Can you work these out from the model? Positions are in its coordinate system, mm. A direction names the side the tool comes from. Coordinates: 2 decimals unless noted, no trailing zeros. Order: outer loops, then holes, each group sorted by start corner. A loop starts at its lowest first (then second) coordinate and runs counter-clockwise, first axis right, second up. Notation, with made-up numbers: M 29,89.5 L 53,89.5 A19 cw 53,98.5 Z; hole C 77.25,-21.75 d9. An arc over 180 degrees is marked long. Answer as a JSON object with one key per item and string values.
from build123d import *

# Parameters (mm, degrees)
BOSS_EXTRUDE1_DEPTH = 6.35
SKETCH2_W           = 88.9
SKETCH2_H           = 6.35
BOSS_EXTRUDE2_DEPTH = 6.35
FILLET1_R           = 2.54
BOSS_EXTRUDE3_DEPTH = 6.35
SKETCH4_R           = 1.5875
CUT_EXTRUDE1_DEPTH  = 296.803693351


with BuildPart() as part:
    # Sketch1 → Boss-Extrude1 (new body)
    with BuildSketch(Plane(origin=(0, 0, 0), x_dir=(1, 0, 0), z_dir=(0, 1, 0))):
        with BuildLine():
            ThreePointArc((12.7, 0), (0, -12.7), (-12.7, 0))
            Line((-12.7, 0), (-12.7, -279.4))
            Line((-12.7, -279.4), (12.7, -279.4))
            Line((12.7, -279.4), (12.7, 0))
        make_face()
        with BuildLine():
            ThreePointArc((12.7, 0), (0, 12.7), (-12.7, 0))
            Line((-12.7, 0), (12.7, 0))
        make_face()
        with BuildLine():
            Line((12.7, 0), (-12.7, 0))
            ThreePointArc((-12.7, 0), (0, -12.7), (12.7, 0))
        make_face()
    extrude(amount=BOSS_EXTRUDE1_DEPTH)

    # Sketch2 → Boss-Extrude2 (add)
    with BuildSketch(Plane(origin=(0, 6.35, 0), x_dir=(1, 0, 0), z_dir=(0, 1, 0))):
        with Locations((31.75, -282.575)):
            Rectangle(SKETCH2_W, SKETCH2_H)
    extrude(amount=-BOSS_EXTRUDE2_DEPTH)

    # Fillet1
    fillet1_edges = [part.edges().sort_by_distance(p)[0] for p in [
        (12.7, 3.175, 279.4),
    ]]
    fillet(fillet1_edges, radius=FILLET1_R)

    # Sketch3 → Boss-Extrude3 (add)
    with BuildSketch(Plane(origin=(0, 0, 0), x_dir=(-1, 0, 0), z_dir=(0, -1, 0))):
        with BuildLine():
            Line((-7.384124229, 1.213847931), (7.384124229, 1.213847931))
            Line((7.384124229, 1.213847931), (5.698055631, 17.468424552))
            ThreePointArc((5.698055631, 17.468424552), (0, 22.606), (-5.698055631, 17.468424552))
            Line((-5.698055631, 17.468424552), (-7.384124229, 1.213847931))
        make_face()
    extrude(amount=-BOSS_EXTRUDE3_DEPTH)

    # Sketch4 → Cut-Extrude1 (cut, through all)
    with BuildSketch(Plane(origin=(0, 0, 0), x_dir=(-1, 0, 0), z_dir=(0, -1, 0))):
        with Locations(Location((0, 0, 0), (0, 0, 90))):
            Circle(SKETCH4_R)
    extrude(amount=-CUT_EXTRUDE1_DEPTH, mode=Mode.SUBTRACT)


solid = part.part
Item 1: I want a section at C-C, the plane x = 64.5. Write out the boundary of the cut face in (y, z), plus the area to 3 significant figures.
Answers follow:
{"outline": "M 0,279.4 L 6.35,279.4 L 6.35,285.75 L 0,285.75 Z", "area": "40.3 mm^2"}
Item 2: Please list where these lines run through material, in increasing order: line 1 (Z direction, x = 61.5, y = 6); line 2 (X direction, y = 1, z = 161); line 3 (Z direction, x = -3.5, y = 5.75).
Answers follow:
{"line 1": "z = 279.4 to 285.75", "line 2": "x = -12.7 to 12.7", "line 3": "z = -21.41 to 285.75"}
Item 3: I'm going to push a flat-ended pin straight in: pin 1 (3 mm diameter, centred on x = 60.5, y = 4.5, fed in from -Z). Where does the tip first touch, or does it pass through?
Answers follow:
{"pin 1": "stops at z = 279.4"}
Item 4: Which directions (+Z, -Z, +X, -X, +Y, -Y) give clear straight access to the entire face, cutting with the end or side of a thin tool? Please do faces 1 (the flat face through (-6.04, 3.13, -14.18)), 2 (the flat face through (45, 3, 279.4)).
Answers follow:
{"face 1": "-Z, -X, +Y, -Y", "face 2": "-Z, +X, +Y, -Y"}
Item 5: I want a section at B-B, the plane z = 56. Write out the boundary of the cut face in (x, y), plus the area to 3 significant figures.
Answers follow:
{"outline": "M -12.7,0 L 12.7,0 L 12.7,6.35 L -12.7,6.35 Z", "area": "161 mm^2"}
